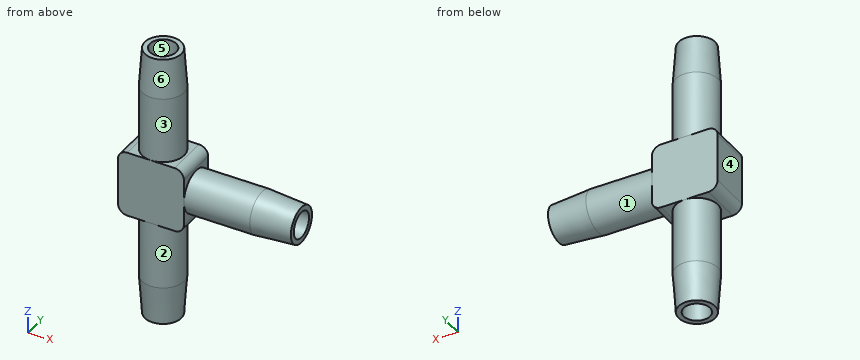
from build123d import *

# Parameters (mm, degrees)
SKETCH1_W               = 10
SKETCH1_H               = 10
BOSS_EXTRUDE1_DEPTH     = 6.4
SKETCH2_R               = 3.2
BOSS_EXTRUDE2_DEPTH     = 10
SKETCH4_R               = 3.2
BOSS_EXTRUDE3_DEPTH     = 10
SKETCH8_R               = 3.2
BOSS_EXTRUDE4_DEPTH     = 6
BOSS_EXTRUDE4_TAPER     = 4
SKETCH10_R              = 3.2
BOSS_EXTRUDE5_DEPTH     = 6
BOSS_EXTRUDE5_TAPER     = 4
FILLET1_R               = 1.4
SKETCH11_R              = 2
CUT_EXTRUDE5_DEPTH      = 48.391560488
CUT_EXTRUDE6_REACH      = 36.029
CUT_EXTRUDE6_END_RADIUS = 2
SKETCH9_R               = 2


with BuildPart() as part:
    # Sketch1 → Boss-Extrude1 (new body)
    with BuildSketch(Plane(origin=(0, 0, 0), x_dir=(1, 0, 0), z_dir=(0, 1, 0))):
        Rectangle(SKETCH1_W, SKETCH1_H)
    extrude(amount=BOSS_EXTRUDE1_DEPTH)

    # Sketch2 → Boss-Extrude2 (add)
    with BuildSketch(Plane.XY.offset(5)):
        with Locations(Location((0, 3.2, 0), (0, 0, 270))):
            Circle(SKETCH2_R)
    boss_extrude2 = extrude(amount=BOSS_EXTRUDE2_DEPTH)

    # Sketch4 → Boss-Extrude3 (add)
    with BuildSketch(Plane(origin=(5, 0, 0), x_dir=(0, 0, -1), z_dir=(1, 0, 0))):
        with Locations(Location((0, 3.2, 0), (0, 0, 270))):
            Circle(SKETCH4_R)
    extrude(amount=BOSS_EXTRUDE3_DEPTH)

    # Sketch8 → Boss-Extrude4 (add)
    with BuildSketch(Plane(origin=(15, 0, 0), x_dir=(0, 0, -1), z_dir=(1, 0, 0))):
        with Locations(Location((0, 3.2, 0), (0, 0, 270))):
            Circle(SKETCH8_R)
    extrude(amount=BOSS_EXTRUDE4_DEPTH, taper=BOSS_EXTRUDE4_TAPER)

    # Sketch10 → Boss-Extrude5 (add)
    with BuildSketch(Plane.XY.offset(15)):
        with Locations(Location((0, 3.2, 0), (0, 0, 270))):
            Circle(SKETCH10_R)
    boss_extrude5 = extrude(amount=BOSS_EXTRUDE5_DEPTH, taper=BOSS_EXTRUDE5_TAPER)

    # Mirror2: Boss-Extrude2, Boss-Extrude5 across plane
    add(boss_extrude2.mirror(Plane.XY))
    add(boss_extrude5.mirror(Plane.XY))

    # Fillet1
    fillet1_edges = [part.edges().sort_by_distance(p)[0] for p in [
        (-5, 3.2, -5),
        (5, 3.2, -5),
        (5, 3.2, 5),
        (-5, 3.2, 5),
    ]]
    fillet(fillet1_edges, radius=FILLET1_R)

    # Sketch11 → Cut-Extrude5 (cut, through all)
    with BuildSketch(Plane.XY.offset(21)):
        with Locations((0, 3.2)):
            Circle(SKETCH11_R)
    extrude(amount=-CUT_EXTRUDE5_DEPTH, mode=Mode.SUBTRACT)

    # Cut-Extrude6: up to this cylinder (the profile starts outside it)
    cut_extrude6_end = Plane(origin=(0, 3.2, 0), z_dir=(0, 0, 1)) * Cylinder(CUT_EXTRUDE6_END_RADIUS, 77.058, mode=Mode.PRIVATE)
    # Sketch9 → Cut-Extrude6 (cut, up to the surface)
    with BuildSketch(Plane(origin=(21, 0, 0), x_dir=(0, 0, -1), z_dir=(1, 0, 0)), mode=Mode.PRIVATE) as cut_extrude6_sk1:
        with Locations((0, 3.2)):
            Circle(SKETCH9_R)
    cut_extrude6_tool1 = extrude(cut_extrude6_sk1.sketch, amount=-CUT_EXTRUDE6_REACH, mode=Mode.PRIVATE) - cut_extrude6_end
    add(cut_extrude6_tool1.solids().sort_by_distance((21, 3.2, 0))[0], mode=Mode.SUBTRACT)


solid = part.part
CAD build for the part. Positions are in the model's coordinates, mm. Face numbers are marked on the shaded views. A direction names the side the tool comes from. Round coordinates to 2 decimals unless told otherwise and drop trailing zeros. Loops run counter-clockwise (first coordinate to the right, second up) from the corner with the lowest first, then second, coordinate; pieces in that order, holes last.
(1) Which spindle directions (+Z, -Z, +X, -X, +Y, -Y) get a long thin tool onto all of the face, cutting with end or side? Do the marked faces 1, 2 and 3. Say none if no direction does.
(2) Wall check: line 1 along Z through (x, y) = (11, 3.2); line 2 along X through (y, z) = (3, 9.5); line 3 along Z through (x, y) = (16, 3). Give the ranges that are in metal, low to high.
(3) Cut at A-A (y = 3.2). State how many separate pieces and enclosed holes the cut face has, plus the area to 3 significant figures.
(4) Drop flat-ended pins along their axis: pin 1 (1.1 mm diameter, centred on x = 1.5, y = 4, fed in from +Z); pin 2 (2 mm diameter, centred on x = 10, y = 3.5, fed in from -Z); pin 3 (3 mm diameter, centred on y = 3.2, z = 0, fed in from +X). Give the stop position or say it passes through.
(5) Cut at C-C (x = 5.5). Give the cut face in (y, z), plus the area to 3 significant figures.
(6) Two-plate mould, pull along X, no slides. Class the marked faces 4, 5 and 6: +X half, -X half, draft (parallel to the pull), parting line (faces both ways), or undercut.
(7) Cut at B-B (z = 12). Give the cut face in (x, y).
Findings below:
1. face 1: +X
1. face 2: -Z
1. face 3: +Z
2. line 1: z = -3.2 to -2, 2 to 3.2
2. line 2: x = -3.19 to -1.99, 1.99 to 3.19
2. line 3: z = -3.12 to -1.99, 1.99 to 3.12
3. separate pieces: 3
3. enclosed holes: 0
3. area: 154 mm2
4. pin 1: stops at z = 21
4. pin 2: stops at z = -3.2
4. pin 3: stops at x = -1.32
5. outline: circle Ø6.4 at (3.2, 0); hole circle Ø4 at (3.2, 0)
5. area: 19.6 mm2
6. face 4: -X half
6. face 5: undercut
6. face 6: parting line
7. outline: circle Ø6.4 at (0, 3.2); hole circle Ø4 at (0, 3.2)
